Part print with two shaded views. Sizes in mm from the minimum x, y, z corner. Round coordinates to 2 decimals unless told otherwise and drop trailing zeros. Loops run counter-clockwise (first coordinate to the right, second up) from the corner with the lowest first, then second, coordinate; pieces in that order, holes last. Notation, with made-up numbers: M 21,67 L 66,67 A22 cw 66,94 Z; hole C 76,15.5 d10. An arc over 180 degrees is marked long. Answer as CSV lines item,"result". Start each with the question number.
Item 1: Drop a flat-ended pin along its axis: pin 1 Ø1 at (x, z) = (185.5, 1) entering from +Y. Give the stop position or say it passes through.
Item 2: Band-saw the part on A-A (z = 5.5). Give the cut face in (x, y) (3 decimals).
Item 3: Wall check: line 1 (Y direction, x = 12.7, z = 1.7); line 2 (Z direction, x = 231.5, y = 17) (3 decimals); line 3 (Y direction, x = 57, z = 5) (3 decimals). Give the ranges that are in metal, low to high.
Item 4: Band-saw the part on B-B (x = 111). Give the cut face in (y, z) (3 decimals).
Item 5: Band-saw the part on C-C (y = 15). Give the cut face in (x, z) (3 decimals), and give its area (3 significant figures).
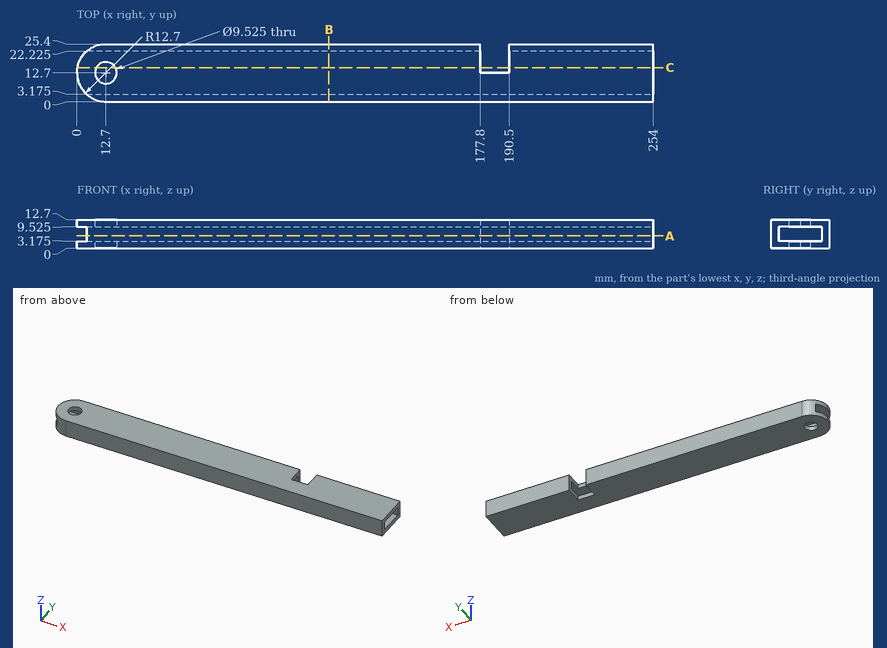
Answer block:
1,pin 1,"stops at y = 12.7"
2,outline,"M 4.3,3.175 A12.7 ccw 12.7,0 L 254,0 L 254,3.175 Z; M 4.3,22.225 L 177.8,22.225 L 177.8,25.4 L 12.7,25.4 A12.7 ccw Z; M 190.5,22.225 L 254,22.225 L 254,25.4 L 190.5,25.4 Z"
3,line 1,"y = 0 to 7.94, 17.46 to 25.4"
3,line 2,"z = 0 to 3.175, 9.525 to 12.7"
3,line 3,"y = 0 to 3.175, 22.225 to 25.4"
4,outline,"M 0,0 L 25.4,0 L 25.4,12.7 L 0,12.7 Z; hole M 3.175,3.175 L 22.225,3.175 L 22.225,9.525 L 3.175,9.525 Z"
5,outline,"M 0.21,0 L 8.53,0 L 8.53,3.175 L 0.21,3.175 Z; M 0.21,9.525 L 8.53,9.525 L 8.53,12.7 L 0.21,12.7 Z; M 16.87,0 L 177.8,0 L 177.8,3.175 L 16.87,3.175 Z; M 16.87,9.525 L 177.8,9.525 L 177.8,12.7 L 16.87,12.7 Z; M 190.5,0 L 254,0 L 254,3.175 L 190.5,3.175 Z; M 190.5,9.525 L 254,9.525 L 254,12.7 L 190.5,12.7 Z"
5,area,"1,480 mm^2"
